Geometry check sheet. Reference: the model listing, model coordinates, mm. A direction names the side the tool comes from. Coordinates: 2 decimals unless noted, no trailing zeros. Loops run counter-clockwise (first coordinate to the right, second up) from the corner with the lowest first, then second, coordinate; pieces in that order, holes last.
Autodesk Inventor part; units mm, degrees
ref_plane "to_screw_XY" through (3, -5.5, 0) normal (1, 0, 0) x (0, 0, -1)
ref_plane "to_screw_YZ" through (3, -5.5, 0) normal (0, 0, -1) x (0, 1, 0)
ref_plane "to_screw_ZX" through (3, -5.5, 0) normal (0, 1, 0) x (1, 0, 0)
sketch "Sketch_1" plane through (0, 0, 0) normal (1, 0, 0) x (0, 1, 0)
  line L0 (0, -5) -> (0, 5)
  line L1 (7.5, 3) -> (3, 3)
  line L2 (3, 3) -> (2.5, 2.5)
  line L3 (2.5, 2.5) -> (2.5, -2.5)
  line L4 (2.5, -2.5) -> (3, -3)
  line L5 (3, -3) -> (7.5, -3)
  line L6 (7.5, -3) -> (8, -2.5)
  line L7 (8, -2.5) -> (8, 2.5)
  line L8 (8, 2.5) -> (7.5, 3)
revolve "Revolution1" add sketch "Sketch_1" angle 360 about axis through (0, 0, -5) along (0, 0, 1)
sketch "Sketch_2" plane through (0, 0, 0) normal (0, 0, 1) x (1, 0, 0)
  line L0 (9.6, -5.5) -> (0.5, -5.5)
  line L1 (0.5, -5.5) -> (0.5, -4.05)
  line L2 (0.5, -4.05) -> (3, -4.05)
  line L3 (3, -4.05) -> (3, -3.05)
  line L4 (3, -3.05) -> (9.6, -3.05)
  line L5 (9.6, -3.05) -> (9.6, -5.5)
  line L6 (9.6, -5.5) -> (0.5, -5.5)
revolve "Revolution2" cut sketch "Sketch_2" angle 360 about axis through (9.6, -5.5, 0) along (1, 0, 0)
sketch "Sketch_3" plane through (0, 0, 0) normal (0, 0, 1) x (1, 0, 0)
  line L0 (-0.5, -5.5) -> (-8, -5.5)
  line L1 (-8, -5.5) -> (-8, -4.4435)
  line L2 (-8, -4.4435) -> (-0.7435, -4.4435)
  line L3 (-0.7435, -4.4435) -> (-0.5, -4.2)
  line L4 (-0.5, -4.2) -> (-0.5, -5.5)
  line L5 (-0.5, -5.5) -> (-8, -5.5)
revolve "Revolution3" cut sketch "Sketch_3" angle 360 about axis through (-0.5, -5.5, 0) along (1, 0, 0)
thread "Thread1"
sketch "Sketch_5" plane through (0, 0, 0) normal (0, 0, 1) x (1, 0, 0)
  line L0 (-0.5, 6) -> (-0.5, -9.6)
  line L1 (-0.5, -9.6) -> (0.5, -9.6)
  line L2 (0.5, -9.6) -> (0.5, 6)
  line L3 (0.5, 6) -> (-0.5, 6)
extrude "Extrusion1" cut sketch "Sketch_5" along normal mid plane 6
ref_plane "to_screw_XY" through (3, -5.5, 0) normal (1, 0, 0) x (0, 0, -1)
ref_plane "to_screw_YZ" through (3, -5.5, 0) normal (0, 0, -1) x (0, 1, 0)
ref_plane "to_screw_ZX" through (3, -5.5, 0) normal (0, 1, 0) x (1, 0, 0)
properties part number "SSCSJ5-6b"
1) Material ranges on probe 1 along Y at (x, z) = (-2.1, 0); probe 2 along Z at (x, y) = (2.35, -5.5); probe 3 along Z at (x, y) = (5, -5.5), recorded low to high.
Data:
probe 1: y = -7.72 to -6.56, -4.44 to -1.36, 1.36 to 7.72
probe 2: z = -3 to -1.45, 1.45 to 3
probe 3: z = -3 to -2.45, 2.45 to 3
2) Section check C-C on x = 2. Count the separate pieces of the cut face and the enclosed holes in it, and give its area (3 significant figures).
Data:
separate pieces: 2
enclosed holes: 1
area: 67.1 mm2
3) Mould release check, pull along Y, two halves, no side actions. Record for faces 1 (the flat face through (0, 6, 0)), 2 (the conical face through (2.64, -0.05, 2.64)), 3 (the cylindrical face through (1.77, -6.95, 0.06)), 4 (the flat face through (3.2, -0.1, -3)): +Y half, -Y half, draft (parallel to the pull), parting line (faces both ways), or undercut.
Data:
face 1: -Y half
face 2: undercut
face 3: undercut
face 4: draft
4) Section check D-D on z = -1.75. Record the cut outline in (x, y).
Data:
outline: (-0.5, -7.98) - (-0.5, -2.45) arc R2.5 cw to (-0.5, 2.45) - (-0.5, 6) - (0.5, 6) - (0.5, 2.45) arc R2.5 cw to (0.5, -2.45) - (0.5, -7.98) arc R8 ccw to (3.46, -7.21) - (3, -7.21) - (3, -3.79) - (7.05, -3.79) arc R8 ccw (long way) to start
5) Section check B-B on z = 0. Record the cut outline in (x, y).
Data:
outline: (-6.65, -4.44) - (-0.74, -4.44) - (-0.5, -4.2) - (-0.5, -2.45) arc R2.5 cw to (-0.5, 2.45) - (-0.5, 6) - (0.5, 6) - (0.5, 2.45) arc R2.5 cw to (0.5, -2.45) - (0.5, -4.05) - (3, -4.05) - (3, -3.05) - (7.4, -3.05) arc R8 ccw (long way) to start; (-4.58, -6.56) arc R8 ccw to (-0.5, -7.98) - (-0.5, -6.8) - (-0.74, -6.56) - close; (0.5, -7.98) arc R8 ccw to (3, -7.42) - (3, -6.95) - (0.5, -6.95) - close
6) Access from +Z, -Z, +X, -X, +Y, -Y to the whole of each face (thin tool, end or side, straight path). Record for faces 5 (the cylindrical face through (-2.5, 0, 0)), 6 (the flat face through (0.5, -4, -1)), 7 (the conical face through (-2.64, -0.05, -2.64)).
Data:
face 5: +Z, -Z
face 6: +Z, -Z, -Y
face 7: -Z
7) Section check A-A on y = 0. Record the cut outline in (x, z), and give its area (3 significant figures).
Data:
outline: (-8, -2.5) - (-7.5, -3) - (-3, -3) - (-2.5, -2.5) - (-2.5, 2.5) - (-3, 3) - (-7.5, 3) - (-8, 2.5) - close; (2.5, -2.5) - (3, -3) - (7.5, -3) - (8, -2.5) - (8, 2.5) - (7.5, 3) - (3, 3) - (2.5, 2.5) - close
area: 65.0 mm2
8) Depth check by flat-ended pin: pin 1 (3 mm diameter, centred on y = -5.5, z = -0.5, fed in from -X); pin 2 (2.5 mm diameter, centred on y = -5.5, z = 0, fed in from -X); pin 3 (1.1 mm diameter, centred on y = 5, z = -1, fed in from +X). Enter the tip coordinate at first touch or a pass-through.
Data:
pin 1: stops at x = -6.93
pin 2: stops at x = -6.78
pin 3: stops at x = 6.65
